Answer from the drawing. Dimensions are ordinates in mm from the lowest x, y and z of the part. A direction names the side the tool comes from. Coordinates: 2 decimals unless noted, no trailing zeros. Order: outer loops, then holes, each group sorted by start corner. A loop starts at its lowest first (then second) coordinate and runs counter-clockwise, first axis right, second up. Notation, with made-up numbers: (57.5, 24) - (113.5, 24) arc R21 cw to (113.5, 40) - close; hole circle Ø3 at (86, -34.75). An arc over 180 degrees is marked (long way). Use a Markdown table: item, result. Add a question column.
Item 1: The part is cut by section C-C, the plane x = 36. Give the vertices of the cut face in (y, z).
Item 2: The mould has two halves that part along Y. Classify the marked faces 3, 4 and 5: released by +Y, released by -Y, zero draft, split by the parting line, or undercut.
Item 3: For the marked faces 1 and 2, determine the directions among +Z, -Z, +X, -X, +Y, -Y from which every point of the face is accessible in a straight line to the end or side of a thin tool.
Item 4: Flat-ended cylindrical pins translate along their axes: P1, Ø6, axis at x = 12, y = 38.5, coming from the -Z side; P2, Ø4, axis at x = 47.5, z = 30, coming from the +Y side; P3, Ø1.5, axis at x = 9.5, y = 22.5, coming from the -Z side. Find the tip coordinate at first contact, or state that the pin passes through.
Item 5: Find the intervals of material crossed by line 1 along X through (y, z) = (33.5, 37); line 2 along Z through (x, y) = (51.5, 32) (1 decimal); line 3 along Y through (x, z) = (36, 30), in increasing order.
Item 6: The part is cut by section B-B, the plane z = 30. Give the vertices of the cut face in (x, y).
Item 7: The part is cut by section A-A, the plane x = 47. Give the vertices of the cut face in (y, z), then the cut area to 3 significant figures.
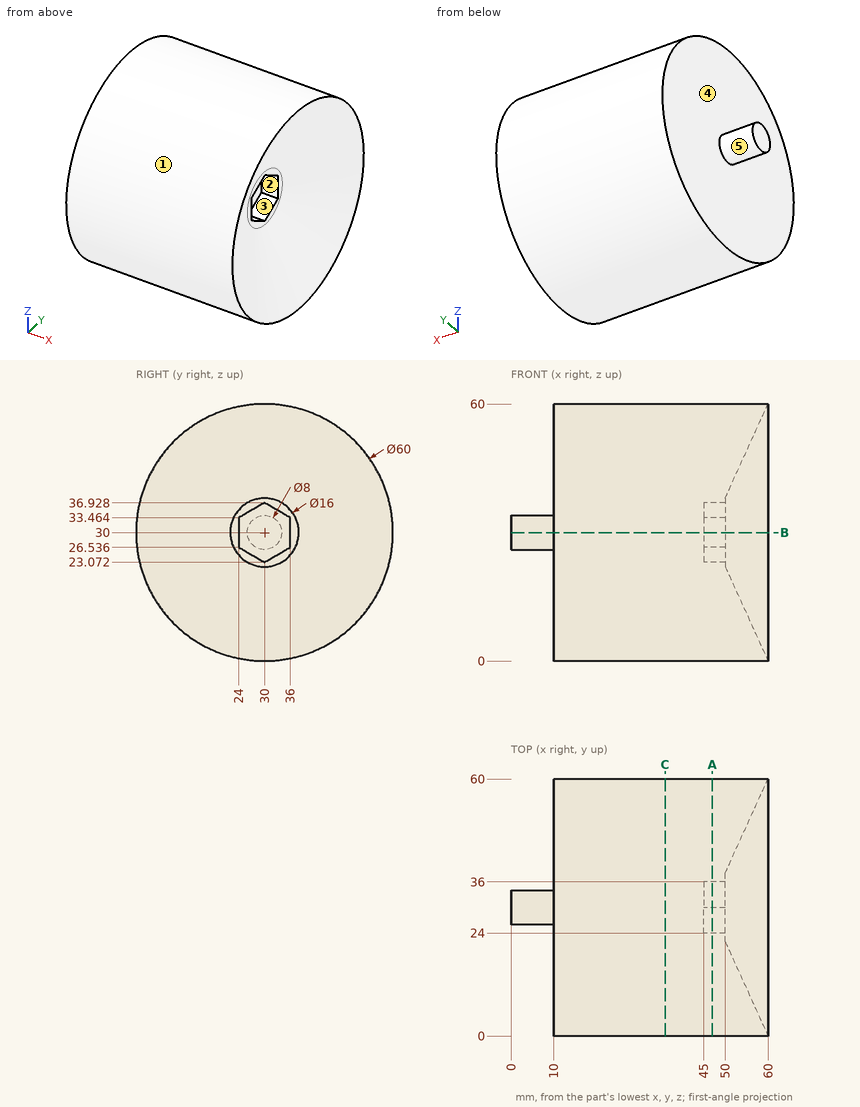
Solution:
| question | item | result |
|---|---|---|
| 1 | outline | circle Ø60 at (30, 30) |
| 2 | face 3 | undercut |
| 2 | face 4 | zero draft |
| 2 | face 5 | split by the parting line |
| 3 | face 1 | +X, -X |
| 3 | face 2 | +X |
| 4 | P1 | stops at z = 0.51 |
| 4 | P2 | stops at y = 60 |
| 4 | P3 | stops at z = 0.81 |
| 5 | line 1 | x = 10 to 50 |
| 5 | line 2 | z = 0.1 to 18.9, 41.1 to 59.9 |
| 5 | line 3 | y = 0 to 60 |
| 6 | outline | (0, 26) - (10, 26) - (10, 0) - (60, 0) - (50, 22) - (50, 24) - (45, 24) - (45, 36) - (50, 36) - (50, 38) - (60, 60) - (10, 60) - (10, 34) - (0, 34) - close |
| 7 | outline | circle Ø60 at (30, 30); hole (24, 26.54) - (30, 23.07) - (36, 26.54) - (36, 33.46) - (30, 36.93) - (24, 33.46) - close |
| 7 | area | 2,700 mm2 |
